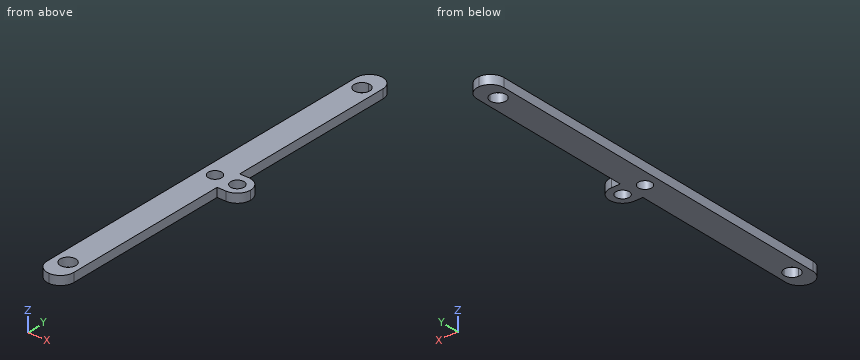
from build123d import *

# Parameters (mm, degrees)
F0_W     = 6
F0_H     = 88
F1_DEPTH = 2
F2_R     = 1.5
F3_DEPTH = 2
F5_DEPTH = 5
F6_R     = 1.5
F7_DEPTH = 2
F8_R     = 2.99999


# Not quite as in the source:
# - a fillet or chamfer is up to 0.001 mm smaller than in the source, because OpenCascade refuses the exact size


with BuildPart() as f1:
    # F0 (on Top) → F1 (new body)
    with BuildSketch(Plane.XY):
        Rectangle(F0_W, F0_H)
    extrude(amount=F1_DEPTH)

    # F2 (on face) → F3 (cut, through all)
    with BuildSketch(Plane.XY.offset(2)):
        Circle(F2_R)
        with BuildLine():
            ThreePointArc((0, 40.75), (-1.2374368671, 37.7625631329), (1.75, 39))
            ThreePointArc((1.75, 39), (1.2374368671, 40.2374368671), (0, 40.75))
        make_face()
        with BuildLine():
            ThreePointArc((0, -40.75), (1.2374368671, -40.2374368671), (1.75, -39))
            ThreePointArc((1.75, -39), (-1.2374368671, -37.7625631329), (0, -40.75))
        make_face()
    extrude(amount=-F3_DEPTH, mode=Mode.SUBTRACT)

    # F4 (on face) → F5 (join)
    with BuildSketch(Plane.YZ.offset(3)):
        Polygon((3, 2), (0, 2), (-3, 2), (-3, 0), (0, 0), (3, 0), align=None)
    extrude(amount=F5_DEPTH)

    # F6 (on face) → F7 (cut, through all)
    with BuildSketch(Plane.XY.offset(2)):
        with Locations((5.0139404441, 0)):
            Circle(F6_R)
    extrude(amount=-F7_DEPTH, mode=Mode.SUBTRACT)

    # F8 (radius 3 in the source; OpenCascade refuses exactly that, so slightly less here)
    f8_edges = [f1.edges().sort_by_distance(p)[0] for p in [
        (-3, -44, 1),
        (3, -44, 1),
        (3, 44, 1),
        (-3, 44, 1),
        (8, -3, 1),
        (8, 3, 1),
    ]]
    fillet(f8_edges, radius=F8_R)


solid = f1.part
The listing builds one solid part. Answer for the finished solid, in the listing's coordinates (mm). Coordinates: 2 decimals unless noted, no trailing zeros. Write each loop counter-clockwise with the first axis right and the second up, starting at its lowest first coordinate (ties: lowest second). Pieces come first, ordered by that corner, then holes. Notation, with made-up numbers: M -10.75,73.5 L 33.25,73.5 A8 cw 33.25,87.5 Z; hole C -7,21.5 d10. An arc over 180 degrees is marked long. Write each question's results on one line, items separated by ' | '.
Item 1: The part is cut by section B-B on y = -23. Determine the outline of the cut face in (x, z), and give its area (3 significant figures).
Answer below:
outline: M -3,0 L 3,0 L 3,2 L -3,2 Z | area: 12.0 mm2
Item 2: The part is cut by section A-A on z = 1.7. State how many separate pieces and enclosed holes the cut face has, and give its area (3 significant figures).
Answer below:
separate pieces: 1 | enclosed holes: 4 | area: 513 mm2
Item 3: Consider probe 1 along Y at (x, z) = (-1, 1.2); probe 2 along Y at (x, z) = (0.5, 0.55); probe 3 along X at (y, z) = (-39, 1.3). Determine where each line is inside the solid, lowest interval first. Write a range as [from, to].
Answer below:
probe 1: [-43.83, -40.44], [-37.56, -1.12], [1.12, 37.56], [40.44, 43.83] | probe 2: [-43.96, -40.68], [-37.32, -1.41], [1.41, 37.32], [40.68, 43.96] | probe 3: [-3, -1.75], [1.75, 3]
Item 4: Given P1, Ø2.5, axis at x = 5.01, y = 0, coming from the +Z side; P2, Ø0.6, axis at y = -23, z = 1, coming from the +X side, each flat-ended and moving along its own axis, determine where each tip first touches the part or whether it passes through.
Answer below:
P1: through | P2: x = 3
